Verification items for the finished model (mm, model axes). Face numbers are marked on the shaded views. A direction names the side the tool comes from. Give positions to 0.01 mm unless a question says otherwise; leave off trailing zeros. Write each loop counter-clockwise with the first axis right and the second up, starting at its lowest first coordinate (ties: lowest second). Pieces come first, ordered by that corner, then holes. Notation, with made-up numbers: (66.25, 40.25) -> (122.25, 40.25) arc R28 ccw to (122.25, 78.25) -> close; hole circle Ø7 at (-40, 81). An arc over 180 degrees is marked (long way). Use one line per item in the form item = value. Start each with the question number.
(1) Section check A-A, the plane z = 32.5. Record the cut outline in (x, y), plus the area to 3 significant figures.
(2) Section check C-C, the plane x = 12.9. Record the cut outline in (y, z), plus the area to 3 significant figures.
(3) Scan lines: L1, parallel to Y at x = 20.75, z = 22; L2, parallel to Y at x = 12.9, z = 3; L3, parallel to X at y = 4, z = 29.5. Record each from-to range of solid material in increasing order.
(4) Set-up check for the marked faces 1 and 2: record each of +Z, -Z, +X, -X, +Y, -Y from which the full face is reachable in a straight line by a thin tool's end or side.
(5) Release check for a two-part mould opening along X. For the marked faces 3, 4 and 5 record: pulls with the +X half, pulls with the -X half, needs draft (parallel to the pull), parting line crosses it, or undercut.
(6) Section check B-B, the plane y = 3.6. Record the cut outline in (x, z).
(7) Depth check by flat-ended pin: pin 1 Ø3 at (x, y) = (13.5, 3) entering from -Z; pin 2 Ø1 at (x, y) = (16.5, 4) entering from +Z; pin 3 Ø3 at (x, z) = (3, 26) entering from -Y. Enter the tip coordinate at first touch or a pass-through.
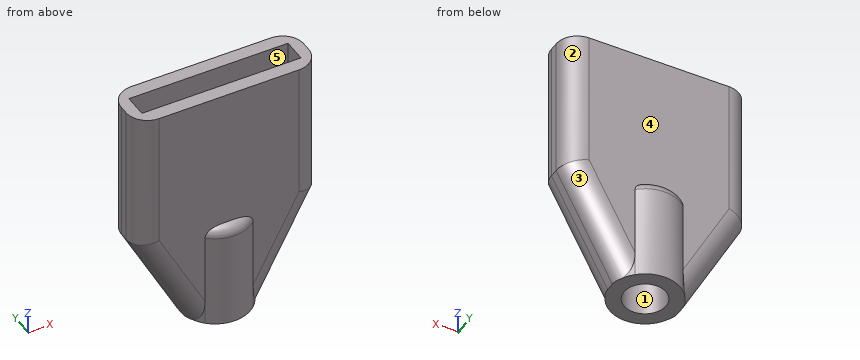
from build123d import *

# Parameters (mm, degrees)
SKETCH1_W           = 25.8
SKETCH1_H           = 35
BOSS_EXTRUDE1_DEPTH = 7.2
SKETCH3_W           = 22.5
SKETCH3_H           = 3.3
CUT_EXTRUDE1_DEPTH  = 20.5
BOSS_EXTRUDE2_DEPTH = 14.9
SKETCH6_R           = 2.95
CUT_EXTRUDE3_DEPTH  = 13.5
FILLET1_R           = 1.4
FILLET2_R           = 1.4
CUT_EXTRUDE4_DEPTH  = 13.5
FILLET5_R           = 3


with BuildPart() as part:
    # Sketch1 → Boss-Extrude1 (new body)
    with BuildSketch(Plane(origin=(0, 0, 0), x_dir=(1, 0, 0), z_dir=(0, 1, 0))):
        with Locations((12.9, -17.5)):
            Rectangle(SKETCH1_W, SKETCH1_H)
    extrude(amount=BOSS_EXTRUDE1_DEPTH)

    # Sketch3 → Cut-Extrude1 (cut)
    with BuildSketch(Plane.XY.offset(35)):
        with Locations((12.9, 3.6)):
            Rectangle(SKETCH3_W, SKETCH3_H)
    extrude(amount=-CUT_EXTRUDE1_DEPTH, mode=Mode.SUBTRACT)

    # Sketch5 → Boss-Extrude2 (add)
    with BuildSketch(Plane(origin=(0, 0, 0), x_dir=(-1, 0, 0), z_dir=(0, 0, -1))):
        with BuildLine():
            Line((-16.297425496, 7.2), (-12.9, 7.2))
            Line((-12.9, 7.2), (-9.502574504, 7.2))
            ThreePointArc((-9.502574504, 7.2), (-12.9, 8.55), (-16.297425496, 7.2))
        make_face()
        with BuildLine():
            Line((-9.502574504, 0), (-12.9, 0))
            Line((-12.9, 0), (-16.297425496, 0))
            ThreePointArc((-16.297425496, 0), (-12.9, -1.35), (-9.502574504, 0))
        make_face()
    extrude(amount=-BOSS_EXTRUDE2_DEPTH)

    # Sketch6 → Cut-Extrude3 (cut)
    with BuildSketch(Plane(origin=(0, 0, 0), x_dir=(-1, 0, 0), z_dir=(0, 0, -1))):
        with Locations((-12.9, 3.6)):
            Circle(SKETCH6_R)
    extrude(amount=-CUT_EXTRUDE3_DEPTH, mode=Mode.SUBTRACT)

    # Fillet1
    # the kernel refuses this fillet: 1.4 mm, written as the material it takes off along each edge
    with BuildSketch(Plane(origin=(12.9, 3.6, 14.9), x_dir=(-0.9942803452588228, 0.10680166212187986, 0), z_dir=(-0.10680166212187986, -0.9942803452588228, 0))) as fillet1_piece_1_section:
        with BuildLine():
            CenterArc((4.95 - FILLET1_R, FILLET1_R), FILLET1_R, 270, 90)
            Line((4.95 - FILLET1_R, 0), (4.95, 0))
            Line((4.95, 0), (4.95, FILLET1_R))
        make_face()
    fillet1_piece_1 = revolve(axis=Axis((12.9, 3.6, 14.9), (0, 0, -1)), revolution_arc=167.738044053, mode=Mode.PRIVATE)
    fillet1_piece_1 = split(fillet1_piece_1, bisect_by=Plane(origin=(12.9, 7.2, 14.482271144), z_dir=(0, 1, 0)), keep=Keep.TOP, mode=Mode.PRIVATE)
    add(fillet1_piece_1, mode=Mode.SUBTRACT)

    # Fillet2
    # the kernel refuses this fillet: 1.4 mm, written as the material it takes off along each edge
    with BuildSketch(Plane(origin=(12.9, 3.6, 14.9), x_dir=(0.9942803452588191, -0.10680166212191289, 0), z_dir=(0.10680166212191289, 0.9942803452588191, 0))) as fillet2_piece_1_section:
        with BuildLine():
            CenterArc((4.95 - FILLET2_R, FILLET2_R), FILLET2_R, 270, 90)
            Line((4.95 - FILLET2_R, 0), (4.95, 0))
            Line((4.95, 0), (4.95, FILLET2_R))
        make_face()
    fillet2_piece_1 = revolve(axis=Axis((12.9, 3.6, 14.9), (0, 0, -1)), revolution_arc=167.738044053, mode=Mode.PRIVATE)
    fillet2_piece_1 = split(fillet2_piece_1, bisect_by=Plane(origin=(12.9, 0, 14.482271144), z_dir=(0, -1, 0)), keep=Keep.TOP, mode=Mode.PRIVATE)
    add(fillet2_piece_1, mode=Mode.SUBTRACT)

    # Sketch7 → Cut-Extrude4 (cut)
    with BuildSketch(Plane(origin=(0, 0, 0), x_dir=(-1, 0, 0), z_dir=(0, -1, 0))):
        Polygon((-17.85, 0), (-25.8, 0), (-25.8, -14.9), align=None)
        Polygon((0, -14.9), (0, 0), (-7.95, 0), align=None)
    extrude(amount=-CUT_EXTRUDE4_DEPTH, mode=Mode.SUBTRACT)

    # Fillet5
    # the kernel refuses this fillet: 3 mm, written as the material it takes off along each edge
    with BuildSketch(Plane(origin=(25.8, 7.2, 7.4), x_dir=(-1, 0, 0), z_dir=(0, 0, 1)), Plane(origin=(0, 7.2, 42.5), x_dir=(1, 0, 0), z_dir=(0, 0, -1))) as fillet5_piece_1:
        with BuildLine():
            CenterArc((FILLET5_R, FILLET5_R), FILLET5_R, 180, 90)
            Line((0, FILLET5_R), (0, 0))
            Line((0, 0), (FILLET5_R, 0))
        make_face()
    extrude(amount=35.1, mode=Mode.SUBTRACT)
    with BuildSketch(Plane(origin=(25.8, 0, 7.4), x_dir=(-1, 0, 0), z_dir=(0, 0, 1)), Plane(origin=(0, 0, 42.5), x_dir=(1, 0, 0), z_dir=(0, 0, -1))) as fillet5_piece_2:
        with BuildLine():
            CenterArc((FILLET5_R, -FILLET5_R), FILLET5_R, 90, 90)
            Line((0, -FILLET5_R), (0, 0))
            Line((0, 0), (FILLET5_R, 0))
        make_face()
    extrude(amount=35.1, mode=Mode.SUBTRACT)
    with BuildSketch(Plane(origin=(29.33056421, 7.2, 21.517032293), x_dir=(0, -1, 0), z_dir=(-0.4707418946375641, 0, -0.8822709723395848))) as fillet5_piece_3_section:
        with BuildLine():
            CenterArc((FILLET5_R, FILLET5_R), FILLET5_R, 180, 90)
            Line((0, FILLET5_R), (0, 0))
            Line((0, 0), (FILLET5_R, 0))
        make_face()
    fillet5_piece_3 = extrude(amount=31.88823555, mode=Mode.PRIVATE)
    fillet5_piece_3 = fillet5_piece_3 - Plane(origin=(12.9, 3.6, 8.289630093), x_dir=(-0.6863485850246219, 0.7272727272727194, 0), z_dir=(0, 0, -1)) * Cylinder(4.95, 76, mode=Mode.PRIVATE)
    add(fillet5_piece_3, mode=Mode.SUBTRACT)
    with BuildSketch(Plane(origin=(29.33056421, 0, 21.517032293), x_dir=(-0.8822709723395848, 0, 0.4707418946375641), z_dir=(-0.4707418946375641, 0, -0.8822709723395848))) as fillet5_piece_4_section:
        with BuildLine():
            CenterArc((FILLET5_R, FILLET5_R), FILLET5_R, 180, 90)
            Line((0, FILLET5_R), (0, 0))
            Line((0, 0), (FILLET5_R, 0))
        make_face()
    fillet5_piece_4 = extrude(amount=31.88823555, mode=Mode.PRIVATE)
    fillet5_piece_4 = fillet5_piece_4 - Plane(origin=(12.9, 3.6, 8.289627813), x_dir=(0.6863485850245981, -0.727272727272742, 0), z_dir=(0, 0, -1)) * Cylinder(4.95, 76, mode=Mode.PRIVATE)
    add(fillet5_piece_4, mode=Mode.SUBTRACT)
    with BuildSketch(Plane(origin=(11.48056421, 7.2, -6.617032293), x_dir=(0.8822709723395851, 0, 0.4707418946375639), z_dir=(-0.4707418946375639, 0, 0.882270972339585))) as fillet5_piece_5_section:
        with BuildLine():
            CenterArc((FILLET5_R, -FILLET5_R), FILLET5_R, 90, 90)
            Line((0, -FILLET5_R), (0, 0))
            Line((0, 0), (FILLET5_R, 0))
        make_face()
    fillet5_piece_5 = extrude(amount=31.88823555, mode=Mode.PRIVATE)
    fillet5_piece_5 = fillet5_piece_5 - Plane(origin=(12.9, 3.6, 8.289627632), x_dir=(-0.6863485850246219, 0.7272727272727194, 0), z_dir=(0, 0, -1)) * Cylinder(4.95, 76, mode=Mode.PRIVATE)
    add(fillet5_piece_5, mode=Mode.SUBTRACT)
    with BuildSketch(Plane(origin=(11.48056421, 0, -6.617032293), x_dir=(0.8822709723395851, 0, 0.4707418946375639), z_dir=(-0.4707418946375639, 0, 0.882270972339585))) as fillet5_piece_6_section:
        with BuildLine():
            CenterArc((FILLET5_R, FILLET5_R), FILLET5_R, 180, 90)
            Line((0, FILLET5_R), (0, 0))
            Line((0, 0), (FILLET5_R, 0))
        make_face()
    fillet5_piece_6 = extrude(amount=31.88823555, mode=Mode.PRIVATE)
    fillet5_piece_6 = fillet5_piece_6 - Plane(origin=(12.9, 3.6, 8.289629174), x_dir=(0.6863485850245981, -0.727272727272742, 0), z_dir=(0, 0, -1)) * Cylinder(4.95, 76, mode=Mode.PRIVATE)
    add(fillet5_piece_6, mode=Mode.SUBTRACT)


solid = part.part
Completed:
q1.outline = (0, 3) arc R3 ccw to (3, 0) -> (22.8, 0) arc R3 ccw to (25.8, 3) -> (25.8, 4.2) arc R3 ccw to (22.8, 7.2) -> (3, 7.2) arc R3 ccw to (0, 4.2) -> close; hole (1.65, 1.95) -> (24.15, 1.95) -> (24.15, 5.25) -> (1.65, 5.25) -> close
q1.area = 104 mm²
q2.outline = (-1.35, 0) -> (0.65, 0) -> (0.65, 13.5) -> (6.55, 13.5) -> (6.55, 0) -> (8.55, 0) -> (8.55, 13.5) arc R1.4 ccw to (7.2, 14.9) -> (7.2, 35) -> (5.25, 35) -> (5.25, 14.5) -> (1.95, 14.5) -> (1.95, 35) -> (0, 35) -> (0, 14.9) arc R1.4 ccw to (-1.35, 13.5) -> close
q2.area = 144 mm²
q3.L1 = 0 to 1.95, 5.25 to 7.2
q3.L2 = -1.35 to 0.65, 6.55 to 8.55
q3.L3 = 0 to 1.65, 24.15 to 25.8
q4.face_1 = -Z
q4.face_2 = +Z, -Z, +X, +Y
q5.face_3 = pulls with the +X half
q5.face_4 = needs draft
q5.face_5 = undercut
q6.outline = (0, 14.9) -> (7.95, 0) -> (9.95, 0) -> (9.95, 13.5) -> (15.85, 13.5) -> (15.85, 0) -> (17.85, 0) -> (25.8, 14.9) -> (25.8, 35) -> (24.15, 35) -> (24.15, 14.5) -> (1.65, 14.5) -> (1.65, 35) -> (0, 35) -> close
q7.pin_1 = 13.5
q7.pin_2 = 14.5
q7.pin_3 = 0
